from build123d import *

# Parameters (mm, degrees)
SKETCH_1_R      = 1.5
EXTRUDE_1_DEPTH = 5


with BuildPart() as part:
    # 草圖1 → 填料-伸長1 (new body)
    with BuildSketch(Plane(origin=(0, 0, 0), x_dir=(1, 0, 0), z_dir=(0, 1, 0))):
        with BuildLine():
            Line((-20, -1.732050808), (-14.090413659, -5.143952072))
            ThreePointArc((-14.090413659, -5.143952072), (0, -15), (14.090413659, -5.143952072))
            Line((14.090413659, -5.143952072), (20, -1.732050808))
            ThreePointArc((20, -1.732050808), (21, 0), (20, 1.732050808))
            Line((20, 1.732050808), (14.090413659, 5.143952072))
            ThreePointArc((14.090413659, 5.143952072), (8.597695008, 12.291445828), (0, 15))
            ThreePointArc((0, 15), (-8.597695008, 12.291445828), (-14.090413659, 5.143952072))
            Line((-14.090413659, 5.143952072), (-20, 1.732050808))
            ThreePointArc((-20, 1.732050808), (-21, 0), (-20, -1.732050808))
        make_face()
        with Locations((-17.5, 0)):
            Circle(SKETCH_1_R, mode=Mode.SUBTRACT)
        with Locations((17.5, 0)):
            Circle(SKETCH_1_R, mode=Mode.SUBTRACT)
    extrude(amount=EXTRUDE_1_DEPTH)


solid = part.part
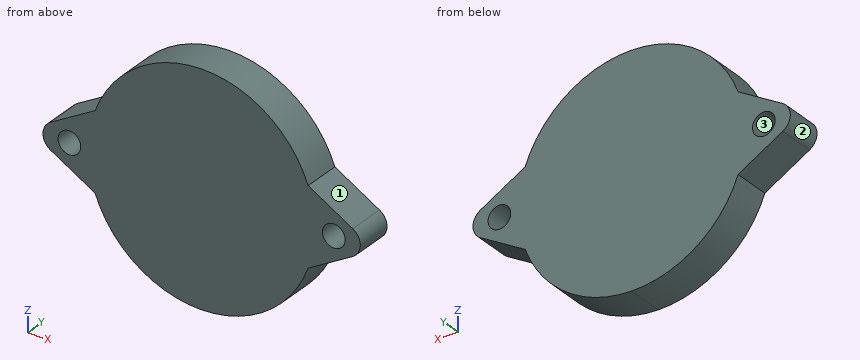
Geometry check sheet. Reference: the model listing, model coordinates, mm. Face numbers are marked on the shaded views. Give positions to 0.01 mm unless a question says otherwise; leave off trailing zeros. Loops run counter-clockwise (first coordinate to the right, second up) from the corner with the lowest first, then second, coordinate; pieces in that order, holes last.
(1) Section check C-C on x = 17.5. Record the cut outline in (y, z).
From the geometry:
outline: (0, -3.18) - (5, -3.18) - (5, -1.5) - (0, -1.5) - close; (0, 1.5) - (5, 1.5) - (5, 3.18) - (0, 3.18) - close
(2) Section check B-B on z = 0. Record the cut outline in (x, y), then the cut area to 3 significant figures.
From the geometry:
outline: (-21, 0) - (-19, 0) - (-19, 5) - (-21, 5) - close; (-16, 0) - (16, 0) - (16, 5) - (-16, 5) - close; (19, 0) - (21, 0) - (21, 5) - (19, 5) - close
area: 180 mm2
(3) Thickness scan on L1, parallel to X at y = 4.4, z = 0.5; L2, parallel to Z at x = 17.5, y = 3.55; L3, parallel to X at y = 1.3, z = 1. Record the ranges inside material, lowest first.
From the geometry:
L1: x = -20.94 to -18.91, -16.09 to 16.09, 18.91 to 20.94
L2: z = -3.18 to -1.5, 1.5 to 3.18
L3: x = -20.73 to -18.62, -16.38 to 16.38, 18.62 to 20.73
(4) Release check for a two-part mould opening along Z. For the marked faces 1, 2 and 3 record: released by +Z, released by -Z, zero draft, split by the parting line, or undercut.
From the geometry:
face 1: released by +Z
face 2: split by the parting line
face 3: undercut
(5) Section check D-D on z = 12. Record the cut outline in (x, y), then the cut area to 3 significant figures.
From the geometry:
outline: (-9, 0) - (9, 0) - (9, 5) - (-9, 5) - close
area: 90.0 mm2
(6) Section check A-A on y = 2.9. Record the cut outline in (x, z), then the cut area to 3 significant figures.
From the geometry:
outline: (-20, -1.73) - (-14.09, -5.14) arc R15 ccw to (14.09, -5.14) - (20, -1.73) arc R2 ccw to (20, 1.73) - (14.09, 5.14) arc R15 ccw to (-14.09, 5.14) - (-20, 1.73) arc R2 ccw to start; hole circle Ø3 at (-17.5, 0); hole circle Ø3 at (17.5, 0)
area: 766 mm2
